Check sheet for the modelled part. Datum: model origin and axes. Units: mm. A direction names the side the tool comes from. Round coordinates to 2 decimals unless told otherwise and drop trailing zeros. Order: outer loops, then holes, each group sorted by start corner. A loop starts at its lowest first (then second) coordinate and runs counter-clockwise, first axis right, second up.
(1) Depth check by flat-ended pin: pin 1 (10 mm diameter, centred on y = 8.5, z = 19.5, fed in from +X); pin 2 (10 mm diameter, centred on x = -13.5, z = -33.5, fed in from +Y); pin 3 (8 mm diameter, centred on x = 18, y = 11.5, fed in from -Z); pin 4 (1 mm diameter, centred on x = 38, z = -15, fed in from +Y). Enter the tip coordinate at first touch or a pass-through.
(2) Sectioned sample at A-A, the plane z = 19. Enter the section's corners in (x, y).
(3) Thickness scan on probe 1 along Y at (x, z) = (-5.5, -7.5); probe 2 along X at (y, z) = (11, -28.5); probe 3 along X at (y, z) = (14.5, 12). Record the ranges inside material, lowest first.
(4) Mould release check, pull along Z, two halves, no side actions. Record for faces 1 (the flat face through (-49, 46.881, -7)), 2 (the flat face through (-18, 2, -40.748)), 3 (the flat face through (-5, 13, 12.592)): released by +Z, released by -Z, zero draft, split by the parting line, or undercut.
(5) Tool access check on faces 4 (the flat face through (-2, -25.4, -7)), 5 (the flat face through (15.722, 13, -34)), 6 (the flat face through (-5, 13, -28.048)). Record the directions out of +Z, -Z, +X, -X, +Y, -Y that give a thin tool (end or side, any length) a straight path to the whole face; none if there is none.
(6) Sectioned sample at C-C, the plane x = 28.5. Enter the section's corners in (y, z), and give its area (3 significant figures).
(7) Sectioned sample at D-D, the plane y = 39.5. Enter the section's corners in (x, z).
(8) Sectioned sample at B-B, the plane y = 2. Enter the section's corners in (x, z), and give its area (3 significant figures).
```python
from build123d import *

# Parameters (mm, degrees)
F0_W     = 144.78
F0_H     = 66.04
F1_DEPTH = 25.4
F2_W     = 88.9
F2_H     = 12.7
F3_DEPTH = 25.4
F4_W     = 48.7939789891
F4_H     = 66.04
F5_DEPTH = 46.88145


with BuildPart() as f1:
    # F0 (on Front) → F1 (new body)
    with BuildSketch(Plane.XZ):
        with Locations((-0.7880558757, -7.7282395214)):
            Rectangle(F0_W, F0_H)
    extrude(amount=F1_DEPTH)

    # F2 (on Front) → F3 (join)
    with BuildSketch(Plane.XZ):
        with Locations((-28.7280558757, -34.3982395214)):
            Rectangle(F2_W, F2_H)
        with Locations((-28.7280558757, 18.9417604786)):
            Rectangle(F2_W, F2_H)
    extrude(amount=-F3_DEPTH)

    # F4 (on Front) → F5 (join)
    with BuildSketch(Plane.XZ):
        with Locations((-48.7810663811, -7.7282395214)):
            Rectangle(F4_W, F4_H)
    extrude(amount=-F5_DEPTH)


solid = f1.part
```
Derived:
1. pin 1: stops at x = 15.72
1. pin 2: stops at y = 25.4
1. pin 3: stops at z = -40.75
1. pin 4: stops at y = 0
2. outline: (-73.18, -25.4) - (71.6, -25.4) - (71.6, 0) - (15.72, 0) - (15.72, 25.4) - (-24.38, 25.4) - (-24.38, 46.88) - (-73.18, 46.88) - close
3. probe 1: y = -25.4 to 0
3. probe 2: x = -73.18 to 15.72
3. probe 3: x = -73.18 to -24.38
4. face 1: zero draft
4. face 2: released by -Z
4. face 3: undercut
5. face 4: +Z, -Z, +X, -X, -Y
5. face 5: +Z, -Z, +X, +Y
5. face 6: +X, +Y
6. outline: (-25.4, -40.75) - (0, -40.75) - (0, 25.29) - (-25.4, 25.29) - close
6. area: 1,680 mm2
7. outline: (-73.18, -40.75) - (-24.38, -40.75) - (-24.38, 25.29) - (-73.18, 25.29) - close
8. outline: (-73.18, -40.75) - (15.72, -40.75) - (15.72, -28.05) - (-24.38, -28.05) - (-24.38, 12.59) - (15.72, 12.59) - (15.72, 25.29) - (-73.18, 25.29) - close
8. area: 4,240 mm2
